Input: part model. Units: mm. Frame: model coordinates. A direction names the side the tool comes from. Give positions to 0.01 mm unless a question says otherwise; leave off trailing zeros. Order: outer loops, then holes, each group sorted by start corner. A loop starts at its lowest first (then second) coordinate and runs counter-clockwise, first axis right, second up. Notation, with made-up numbers: (41.5, 29.25) - (47.5, 29.25) arc R15 cw to (47.5, 39.25) - close; hole circle Ø10 at (-15.75, 86). An arc over 180 degrees is marked (long way). Answer in a Markdown table with one row per item. Add a question column.
1. Section query A-A on y = 13.5. Return loops of the section in (x, z), and give its area (3 significant figures).
2. Ray query, line 1 (X direction, y = -10.5, z = 3.6); line 2 (X direction, y = -17.5, z = 1.8); line 3 (X direction, y = -13.5, z = 3.4). Return the intervals inside material, ascending. Write a range as [from, to].
3. Section query C-C on z = 2.95. Count the separate pieces of the cut face and the enclosed holes in it, and give its area (3 significant figures).
4. Mould query, pull axis Y, two halves, no side actions, for faces 4 (the face through (78, -15, 2)), 5 (the face through (-53, -5, 2)), 6 (the face through (-75, 17, 2)), 7 (the face through (19.7, -0.1, 2.5)). Classes: released by +Y, released by -Y, zero draft, split by the parting line, or undercut.
5. Access query for faces 1 (the face through (-77, -15, 2)), 2 (the face through (-1, 15, 2)), 3 (the face through (-68, -15, 2)). Directions: +Z, -Z, +X, -X, +Y, -Y. A direction counts if a zero-diameter tool reaches every point of the face in a straight line with its end or side. Return the directions, or none.
6. Section query D-D on y = 0. Return loops of the section in (x, z), and give its area (3 significant figures).
7. Contact query for flat-ended pins moving along their axis: pin 1 (2.5 mm diameter, centred on y = -18.5, z = 2.5, fed in from +X); pin 2 (0.6 mm diameter, centred on x = -63, z = 3.5, fed in from +Y). Output: stop coordinate, or through.
8. Section query B-B on x = 23.25. Return loops of the section in (y, z), and give its area (4 significant figures).
```python
from build123d import *

# Parameters (mm, degrees)
SKETCH2_R           = 2.95
SKETCH2_W           = 5
SKETCH2_H           = 5
BOSS_EXTRUDE1_DEPTH = 5


with BuildPart() as part:
    # Sketch2 → Boss-Extrude1 (new body)
    with BuildSketch(Plane.XY):
        Polygon((66.5, 15), (70, 15), (70, 20), (75, 20), (75, 15), (80, 15), (80, -15), (75, -15), (75, -20), (70, -20), (70, -15), (66.5, -15), (66.5, -12), (67.6, -12), (67.6, -9.7), (66.5, -9.7), (66.5, -5), (63.5, -5), (63.5, -9.7), (62.4, -9.7), (62.4, -12), (63.5, -12), (63.5, -15), (60, -15), (60, -20), (55, -20), (55, -15), (-55, -15), (-55, -20), (-60, -20), (-60, -15), (-63.5, -15), (-63.5, -12), (-62.4, -12), (-62.4, -9.7), (-63.5, -9.7), (-63.5, -5), (-66.5, -5), (-66.5, -9.7), (-67.6, -9.7), (-67.6, -12), (-66.5, -12), (-66.5, -15), (-70, -15), (-70, -20), (-75, -20), (-75, -15), (-80, -15), (-80, 15), (-75, 15), (-75, 20), (-70, 20), (-70, 15), (-66.5, 15), (-66.5, 12), (-67.6, 12), (-67.6, 9.7), (-66.5, 9.7), (-66.5, 5), (-63.5, 5), (-63.5, 9.7), (-62.4, 9.7), (-62.4, 12), (-63.5, 12), (-63.5, 15), (-60, 15), (-60, 20), (-55, 20), (-55, 15), (55, 15), (55, 20), (60, 20), (60, 15), (63.5, 15), (63.5, 12), (62.4, 12), (62.4, 9.7), (63.5, 9.7), (63.5, 5), (66.5, 5), (66.5, 9.7), (67.6, 9.7), (67.6, 12), (66.5, 12), align=None)
        with Locations((23.25, 0)):
            Circle(SKETCH2_R, mode=Mode.SUBTRACT)
        with Locations(Location((16.75, 0, 0), (0, 0, 180))):
            Circle(SKETCH2_R, mode=Mode.SUBTRACT)
        with Locations((52.5, 7.5)):
            Rectangle(SKETCH2_W, SKETCH2_H, mode=Mode.SUBTRACT)
        with Locations((52.5, -7.5)):
            Rectangle(SKETCH2_W, SKETCH2_H, mode=Mode.SUBTRACT)
        with Locations((-52.5, 7.5)):
            Rectangle(SKETCH2_W, SKETCH2_H, mode=Mode.SUBTRACT)
        with Locations((-52.5, -7.5)):
            Rectangle(SKETCH2_W, SKETCH2_H, mode=Mode.SUBTRACT)
    extrude(amount=BOSS_EXTRUDE1_DEPTH)


solid = part.part
```
Answer:
| question | item | result |
|---|---|---|
| 1 | outline | (-80, 0) - (-66.5, 0) - (-66.5, 5) - (-80, 5) - close; (-63.5, 0) - (63.5, 0) - (63.5, 5) - (-63.5, 5) - close; (66.5, 0) - (80, 0) - (80, 5) - (66.5, 5) - close |
| 1 | area | 770 mm² |
| 2 | line 1 | x = [-80, -67.6], [-62.4, 62.4], [67.6, 80] |
| 2 | line 2 | x = [-75, -70], [-60, -55], [55, 60], [70, 75] |
| 2 | line 3 | x = [-80, -66.5], [-63.5, 63.5], [66.5, 80] |
| 3 | separate pieces | 1 |
| 3 | enclosed holes | 6 |
| 3 | area | 4,710 mm² |
| 4 | face 4 | released by -Y |
| 4 | face 5 | undercut |
| 4 | face 6 | zero draft |
| 4 | face 7 | undercut |
| 5 | face 1 | +Z, -Z, -X, -Y |
| 5 | face 2 | +Z, -Z, +Y |
| 5 | face 3 | +Z, -Z, -Y |
| 6 | outline | (-80, 0) - (13.8, 0) - (13.8, 5) - (-80, 5) - close; (19.7, 0) - (20.3, 0) - (20.3, 5) - (19.7, 5) - close; (26.2, 0) - (80, 0) - (80, 5) - (26.2, 5) - close |
| 6 | area | 741 mm² |
| 7 | pin 1 | stops at x = 75 |
| 7 | pin 2 | stops at y = 15 |
| 8 | outline | (-15, 0) - (-2.95, 0) - (-2.95, 5) - (-15, 5) - close; (2.95, 0) - (15, 0) - (15, 5) - (2.95, 5) - close |
| 8 | area | 120.5 mm² |
